Input: part model. Units: mm. Frame: model coordinates. Face numbers are marked on the shaded views. Give positions to 0.01 mm unless a question says otherwise; leave off trailing zeros. Order: outer loops, then holes, each group sorted by start corner. A loop starts at its lowest first (then second) coordinate and runs counter-clockwise, first axis right, second up.
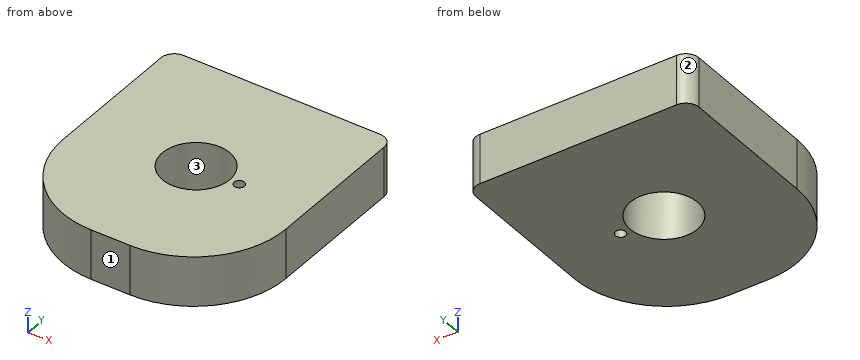
```python
from build123d import *

# Parameters (mm, degrees)
F0_W     = 21.5
F0_H     = 23.8
F0_R     = 0.5
F0_R_2   = 3.25
F1_DEPTH = 4.8
F2_R     = 8.89
F3_R     = 1.27


# Not quite as in the source:
# - a feature of the source that left no trace in its solid (it failed there, or was rolled back) is left out


with BuildPart() as f1:
    # F0 (on Top) → F1 (new body)
    with BuildSketch(Plane.XY):
        with Locations((10.75, 11.9)):
            Rectangle(F0_W, F0_H)
        with Locations((14.9710876867, 11.8254814297)):
            Circle(F0_R, mode=Mode.SUBTRACT)
        with Locations((10.75, 11.9)):
            Circle(F0_R_2, mode=Mode.SUBTRACT)
    extrude(amount=F1_DEPTH)

    # F2
    f2_edges = [f1.edges().sort_by_distance(p)[0] for p in [
        (21.5, 0, 2.4),
        (0, 0, 2.4),
    ]]
    fillet(f2_edges, radius=F2_R)

    # F3
    f3_edges = [f1.edges().sort_by_distance(p)[0] for p in [
        (21.5, 23.8, 2.4),
        (0, 23.8, 2.4),
    ]]
    fillet(f3_edges, radius=F3_R)


solid = f1.part
```
1) Cut plane D-D (y = 5.75). Return the cut outline in (x, z).
2) Cut plane B-B (z = 2.55). Return the cut outline in (x, y).
3) Pull-direction query (Y, two-part tool) for the marked faces 1, 2 and 3; classes: pulls with the +Y half, pulls with the -Y half, needs draft (parallel to the pull), parting line crosses it, or undercut.
4) Cut plane A-A (x = 10.75). Return the cut outline in (y, z).
5) Cut plane C-C (x = 8.25). Return the cut outline in (y, z).
6) Line query: probe 1 along Y at (x, z) = (8, 2.2); probe 2 along X at (y, z) = (13, 0.75); probe 3 along Y at (x, z) = (8.75, 2.3). Output: solid intervals per line, ascending.
Geometry says:
1. outline: (0.57, 0) - (20.93, 0) - (20.93, 4.8) - (0.57, 4.8) - close
2. outline: (0, 8.89) arc R8.89 ccw to (8.89, 0) - (12.61, 0) arc R8.89 ccw to (21.5, 8.89) - (21.5, 22.53) arc R1.27 ccw to (20.23, 23.8) - (1.27, 23.8) arc R1.27 ccw to (0, 22.53) - close; hole circle Ø6.5 at (10.75, 11.9); hole circle Ø1 at (14.97, 11.83)
3. face 1: pulls with the -Y half
3. face 2: pulls with the +Y half
3. face 3: undercut
4. outline: (0, 0) - (8.65, 0) - (8.65, 4.8) - (0, 4.8) - close; (15.15, 0) - (23.8, 0) - (23.8, 4.8) - (15.15, 4.8) - close
5. outline: (0.02, 0) - (9.82, 0) - (9.82, 4.8) - (0.02, 4.8) - close; (13.98, 0) - (23.8, 0) - (23.8, 4.8) - (13.98, 4.8) - close
6. probe 1: y = 0.04 to 10.17, 13.63 to 23.8
6. probe 2: x = 0 to 7.69, 13.81 to 21.5
6. probe 3: y = 0 to 9.34, 14.46 to 23.8
